Work out the finished part from the listing and answer in its coordinate system (mm). A direction names the side the tool comes from. Give positions to 0.01 mm unless a question says otherwise; leave off trailing zeros. Write each loop counter-clockwise with the first axis right and the second up, starting at its lowest first coordinate (ties: lowest second). Pieces come first, ordered by that corner, then holes. Notation, with made-up numbers: (3, 52.5) - (10, 52.5) arc R18 cw to (10, 63.5) - close; hole circle Ø9 at (-24, 41.5). An arc over 180 degrees is marked (long way). Write item = value, one per line.
from build123d import *

# Parameters (mm, degrees)
SKETCH1_W                      = 132.08
SKETCH1_H                      = 161.925
BOSS_EXTRUDE1_DEPTH            = 3.175
FILLET1_R                      = 6.35
TAP_DRILL_FOR_M3X0_5_TAP1_D    = 2.5
SKETCH5_W                      = 82.226471496
SKETCH5_H                      = 7.747
BOSS_EXTRUDE2_DEPTH            = 9.271
TAP_DRILL_FOR_M3X0_5_TAP2_D    = 2.5
CBORE_FOR_M3_SHCS1_D           = 3.4
CBORE_FOR_M3_SHCS1_CBORE_D     = 6.5
CBORE_FOR_M3_SHCS1_CBORE_DEPTH = 3


with BuildPart() as part:
    # Sketch1 → Boss-Extrude1 (new body)
    with BuildSketch(Plane(origin=(0, 0, 0), x_dir=(1, 0, 0), z_dir=(0, 1, 0))):
        Rectangle(SKETCH1_W, SKETCH1_H)
    extrude(amount=BOSS_EXTRUDE1_DEPTH)

    # Fillet1
    fillet1_edges = [part.edges().sort_by_distance(p)[0] for p in [
        (-66.04, 1.5875, -80.9625),
        (66.04, 1.5875, -80.9625),
        (66.04, 1.5875, 80.9625),
        (-66.04, 1.5875, 80.9625),
    ]]
    fillet(fillet1_edges, radius=FILLET1_R)

    # Tap Drill for M3x0.5 Tap1 (through all)
    with Locations(Plane(origin=(0, 3.175, 0), x_dir=(1, 0, 0), z_dir=(0, 1, 0))):
        with Locations((56.515, -75.40625), (56.515, 75.40625)):
            Hole(TAP_DRILL_FOR_M3X0_5_TAP1_D / 2)

    # Sketch5 → Boss-Extrude2 (add)
    with BuildSketch(Plane(origin=(0, 3.175, 0), x_dir=(1, 0, 0), z_dir=(0, 1, 0))):
        with Locations((-14.7701, 0)):
            Rectangle(SKETCH5_W, SKETCH5_H)
    extrude(amount=BOSS_EXTRUDE2_DEPTH)

    # Tap Drill for M3x0.5 Tap2 (through all)
    with Locations(Plane(origin=(0, 12.446, 0), x_dir=(1, 0, 0), z_dir=(0, 1, 0))):
        with Locations((-46.5201, 0), (16.9799, 0)):
            Hole(TAP_DRILL_FOR_M3X0_5_TAP2_D / 2)

    # CBORE for M3 SHCS1 (through all)
    with Locations(Plane(origin=(0, 12.446, 0), x_dir=(1, 0, 0), z_dir=(0, 1, 0))):
        with Locations((4.2799, 0), (-33.8201, 0)):
            CounterBoreHole(CBORE_FOR_M3_SHCS1_D / 2, CBORE_FOR_M3_SHCS1_CBORE_D / 2, CBORE_FOR_M3_SHCS1_CBORE_DEPTH)


solid = part.part
1. Find section B-B, the plane x = -24.5. Give the vertices of the cut face in (y, z) (1 decimal).
Solution:
outline = (0, -81) - (3.2, -81) - (3.2, -3.9) - (12.4, -3.9) - (12.4, 3.9) - (3.2, 3.9) - (3.2, 81) - (0, 81) - close
2. For a pull along X with two mould halves and no side action, classify faces 5 (the flat face through (-1, 0, -1)), 6 (the flat face through (66.04, 2, 1)), 7 (the cylindrical face through (-32.12, 4.66, -0.07)), 8 (the cylindrical face through (-64.23, 1.61, 79.05)) as pulls with the +X half, pulls with the -X half, needs draft (parallel to the pull), parting line crosses it, or undercut.
Solution:
face_5 = needs draft
face_6 = pulls with the +X half
face_7 = undercut
face_8 = pulls with the -X half
3. Find section A-A, the plane y = 5.25. Give the vertices of the cut face in (x, z).
Solution:
outline = (-55.88, -3.87) - (26.34, -3.87) - (26.34, 3.87) - (-55.88, 3.87) - close; hole circle Ø2.5 at (-46.52, 0); hole circle Ø3.4 at (-33.82, 0); hole circle Ø3.4 at (4.28, 0); hole circle Ø2.5 at (16.98, 0)
4. Given pin 1 (4 mm diameter, centred on x = 4.28, z = 0, fed in from +Y); pin 2 (4.5 mm diameter, centred on x = -25.5, y = 6, fed in from +Z); pin 3 (10 mm diameter, centred on x = 28, z = 32, fed in from +Y) (3 decimals); pin 4 (7 mm diameter, centred on x = -34, z = 0, fed in from +Y), each flat-ended and moving along its own axis, determine where each tip first touches the part or whether it passes through.
Solution:
pin_1 = 9.45
pin_2 = 3.87
pin_3 = 3.175
pin_4 = 12.45
5. A tool of negligible diameter and unlimited length cuts with its end or side. For faces 1 (the flat face through (-55.883, 8, 0)), 2 (the cylindrical face through (-37.067, 10.967, -0.143)), 3 (the flat face through (-15, 8, -3.874)), 4 (the flat face through (-15, 8, 3.874)), from which of +Z, -Z, +X, -X, +Y, -Y can it reach the whole face along a straight path? Write none if from no direction.
Solution:
face_1 = +Z, -Z, -X, +Y
face_2 = +Y
face_3 = -Z, +X, -X, +Y
face_4 = +Z, +X, -X, +Y
6. Find section C-C, the plane z = 11. Give the vertices of the cut face in (x, y) (3 decimals), then the cut area to 3 significant figures.
Solution:
outline = (-66.04, 0) - (66.04, 0) - (66.04, 3.175) - (-66.04, 3.175) - close
area = 419 mm^2
7. Straight lines are drawn through the part: line 1 (X direction, y = 7, z = -1.5); line 2 (Y direction, x = -4, z = -28) (3 decimals); line 3 (Z direction, x = 8.5, y = 3.5). For each, find the intervals that lie inside material, in ascending order.
Solution:
line_1 = -55.88 to -34.62, -33.02 to 3.48, 5.08 to 26.34
line_2 = 0 to 3.175
line_3 = -3.87 to 3.87
